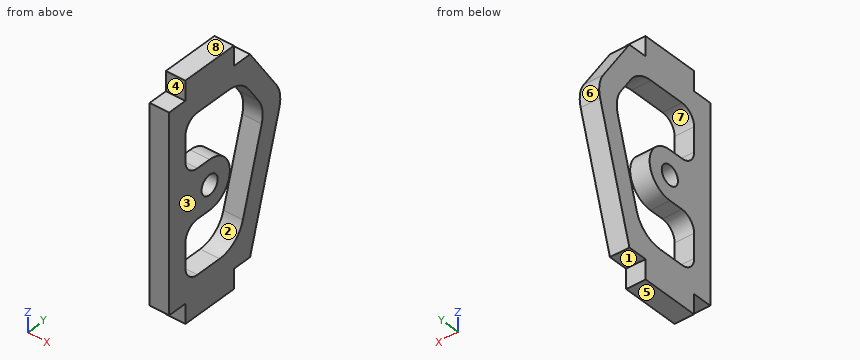
from build123d import *

# Parameters (mm, degrees)
F1_DEPTH = 2
F3_DEPTH = 2
F4_R     = 1
F5_DEPTH = 2.001
F7_DEPTH = 2.001


with BuildPart() as f1:
    # F0 (on Right) → F1 (new body)
    with BuildSketch(Plane.YZ):
        Polygon((-3, 0), (-3, -2), (3, -2), (3, 0), (5, 0), (5, 20), (3, 20), (3, 22), (-3, 22), (-3, 20), (-5, 20), (-5, 0), align=None)
    extrude(amount=F1_DEPTH)

    # F2 (on face) → F3 (join, through all)
    with BuildSketch(Plane.YZ.offset(2)):
        with BuildLine():
            Line((3, 0), (5, 0))
            Line((5, 0), (8.618873, 12.666057))
            ThreePointArc((8.618873, 12.666057), (8.698405, 13.952921), (8.230453, 15.154321))
            Line((8.230453, 15.154321), (5, 20))
            Line((5, 20), (3, 20))
            Line((3, 20), (3, 0))
        make_face()
    extrude(amount=-F3_DEPTH)

    # F4 (on face) → F5 (cut, through all)
    with BuildSketch(Plane.YZ.offset(2)):
        with Locations((0, 10)):
            Circle(F4_R)
    extrude(amount=-F5_DEPTH, mode=Mode.SUBTRACT)

    # F6 (on face) → F7 (cut, through all)
    with BuildSketch(Plane.YZ.offset(2)):
        with BuildLine():
            ThreePointArc((1.228493, 2), (3.035079, 2.604954), (4.113065, 4.175837))
            Line((4.113065, 4.175837), (6.441741, 12.326204))
            ThreePointArc((6.441741, 12.326204), (6.521273, 13.613068), (6.05332, 14.814468))
            Line((6.05332, 14.814468), (4.820232, 16.664101))
            ThreePointArc((4.820232, 16.664101), (3.739655, 17.645024), (2.324081, 18))
            Line((2.324081, 18), (-1.5, 18))
            ThreePointArc((-1.5, 18), (-2.56066, 17.56066), (-3, 16.5))
            Line((-3, 16.5), (-3, 14))
            ThreePointArc((-3, 14), (-2.56066, 12.93934), (-1.5, 12.5))
            Line((-1.5, 12.5), (0, 12.5))
            ThreePointArc((0, 12.5), (2.5, 10), (0, 7.5))
            Line((0, 7.5), (-1.5, 7.5))
            ThreePointArc((-1.5, 7.5), (-2.56066, 7.06066), (-3, 6))
            Line((-3, 6), (-3, 3.5))
            ThreePointArc((-3, 3.5), (-2.56066, 2.43934), (-1.5, 2))
            Line((-1.5, 2), (1.228493, 2))
        make_face()
    extrude(amount=-F7_DEPTH, mode=Mode.SUBTRACT)


solid = f1.part
Geometry: final body of the model. Coordinates: model frame, mm. Face numbers are marked on the shaded views. A direction names the side the tool comes from. Give positions to 0.01 mm unless a question says otherwise; leave off trailing zeros. Write each loop counter-clockwise with the first axis right and the second up, starting at its lowest first coordinate (ties: lowest second). Pieces come first, ordered by that corner, then holes.
(1) Mould query, pull axis Y, two halves, no side actions, for the marked faces 6, 7 and 8. Classes: released by +Y, released by -Y, zero draft, split by the parting line, or undercut.
(2) Cut plane A-A, the plane x = 0.85. Give the number of separate pieces and of enclosed holes in the cut face, then the cut area to 3 significant figures.
(3) Access query for the marked faces 1, 2, 3, 4 and 5. Directions: +Z, -Z, +X, -X, +Y, -Y. A direction counts if a zero-diameter tool reaches every point of the face in a straight line with its end or side. Return the directions, or none.
(4) Ray query, line 1 (Z direction, x = 0.95, y = -4.25); line 2 (Z direction, x = 1.55, y = 2.25); line 3 (Y direction, x = 1.3, z = 11.5). Return the intervals inside material, ascending.
(5) Cut plane B-B, the plane z = 11.25. Return loops of the section in (x, y), then the cut area to 3 significant figures.
(6) Cut plane D-D, the plane y = -3.25. Return loops of the section in (x, z), then the cut area to 3 significant figures.
(7) Cut plane C-C, the plane y = 5.5. Return loops of the section in (x, z).
(8) First-contact query: P1, Ø0.6, axis at x = 1, y = 4, coming from the +Z side; P2, Ø0.6, axis at x = 1, y = 3.5, coming from the -Z side; P3, Ø1, axis at x = 0.5, z = -1, coming from the -Y side; P4, Ø1.2, axis at y = 0, z = 10, coming from the +X side. Flat tips, straight axial feed; report the tip coordinate or a pass-through.
Values follow:
1. face 6: released by +Y
1. face 7: undercut
1. face 8: zero draft
2. separate pieces: 1
2. enclosed holes: 2
2. area: 158 mm2
3. face 1: -Z, +X, -X, +Y
3. face 2: +X, -X
3. face 3: +Z, -Z, +X, +Y, -Y
3. face 4: +Z, +X, -X, -Y
3. face 5: -Z, +X, -X, +Y, -Y
4. line 1: z = 0 to 20
4. line 2: z = -2 to 2.18, 8.91 to 11.09, 18 to 22
4. line 3: y = -5 to 2, 6.21 to 8.29
5. outline: (0, -5) - (2, -5) - (2, 2.17) - (0, 2.17) - close; (0, 6.13) - (2, 6.13) - (2, 8.21) - (0, 8.21) - close
5. area: 18.5 mm2
6. outline: (0, 0) - (2, 0) - (2, 20) - (0, 20) - close
6. area: 40.0 mm2
7. outline: (0, 1.75) - (2, 1.75) - (2, 9.03) - (0, 9.03) - close; (0, 15.64) - (2, 15.64) - (2, 19.25) - (0, 19.25) - close
8. P1: stops at z = 20
8. P2: stops at z = 0
8. P3: stops at y = -3
8. P4: passes through
